Input: part model. Units: mm. Frame: model coordinates. A direction names the side the tool comes from. Round coordinates to 2 decimals unless told otherwise and drop trailing zeros. Write each loop counter-clockwise with the first axis right and the second up, starting at its lowest first coordinate (ties: lowest second). Pieces come first, ordered by that corner, then holes. Notation, with made-up numbers: (12.5, 46.5) -> (54.5, 46.5) arc R11 cw to (54.5, 55.5) -> close; hole circle Ø11 at (60, 10.25). An arc over 180 degrees is marked (long way). Write item = value, one per line. Start each with the question number.
```python
from build123d import *

# Parameters (mm, degrees)
SKETCH1_R           = 11.5
SKETCH1_R_2         = 1.5
SKETCH1_W           = 8.4
SKETCH1_H           = 8.4
BOSS_EXTRUDE1_DEPTH = 8.4


with BuildPart() as part:
    # Sketch1 → Boss-Extrude1 (new body)
    with BuildSketch(Plane(origin=(0, 0, 0), x_dir=(1, 0, 0), z_dir=(0, 1, 0))):
        with BuildLine():
            Line((-34.5, 26), (34.5, 26))
            ThreePointArc((34.5, 26), (36.621320344, 25.121320344), (37.5, 23))
            Line((37.5, 23), (37.5, -26))
            Line((37.5, -26), (23.5, -26))
            Line((23.5, -26), (23.5, -34))
            Line((23.5, -34), (15.5, -34))
            Line((15.5, -34), (15.5, -26))
            Line((15.5, -26), (2, -26))
            Line((2, -26), (2, -21.4))
            Line((2, -21.4), (3.5, -21.4))
            Line((3.5, -21.4), (3.5, -18.4))
            Line((3.5, -18.4), (2.260530911, -18.4))
            ThreePointArc((2.260530911, -18.4), (0, -11.1), (-2.260530911, -18.4))
            Line((-2.260530911, -18.4), (-3.5, -18.4))
            Line((-3.5, -18.4), (-3.5, -21.4))
            Line((-3.5, -21.4), (-2, -21.4))
            Line((-2, -21.4), (-2, -26))
            Line((-2, -26), (-15.5, -26))
            Line((-15.5, -26), (-15.5, -34))
            Line((-15.5, -34), (-23.5, -34))
            Line((-23.5, -34), (-23.5, -26))
            Line((-23.5, -26), (-37.5, -26))
            Line((-37.5, -26), (-37.5, 23))
            ThreePointArc((-37.5, 23), (-36.621320344, 25.121320344), (-34.5, 26))
        make_face()
        with Locations((0, 6)):
            Circle(SKETCH1_R, mode=Mode.SUBTRACT)
        with Locations((15.5, 21.5)):
            Circle(SKETCH1_R_2, mode=Mode.SUBTRACT)
        with Locations((-15.5, 21.5)):
            Circle(SKETCH1_R_2, mode=Mode.SUBTRACT)
        with Locations((15.5, -9.5)):
            Circle(SKETCH1_R_2, mode=Mode.SUBTRACT)
        with Locations((-15.5, -9.5)):
            Circle(SKETCH1_R_2, mode=Mode.SUBTRACT)
        with Locations((-30.1, 2)):
            Circle(SKETCH1_R_2, mode=Mode.SUBTRACT)
        with Locations((30.1, 2)):
            Circle(SKETCH1_R_2, mode=Mode.SUBTRACT)
        with Locations((-30.1, 14.2)):
            Rectangle(SKETCH1_W, SKETCH1_H, mode=Mode.SUBTRACT)
        with Locations((-30.1, -9.8)):
            Rectangle(SKETCH1_W, SKETCH1_H, mode=Mode.SUBTRACT)
        with Locations((30.1, -9.8)):
            Rectangle(SKETCH1_W, SKETCH1_H, mode=Mode.SUBTRACT)
        with Locations((30.1, 14.2)):
            Rectangle(SKETCH1_W, SKETCH1_H, mode=Mode.SUBTRACT)
    extrude(amount=BOSS_EXTRUDE1_DEPTH)


solid = part.part
```
1. Section D-D (z = -21.5). Output: boundary loops of the cut face in (x, y).
2. Section A-A (z = 27.5). Output: boundary loops of the cut face in (x, y), then the cut area to 3 significant figures.
3. Reachability of faces 1 (the flat face through (30, 4, 14)), 2 (the flat face through (23.5, 4, 30)), 3 (the flat face through (9, 4, 26)) from +Z, -Z, +X, -X, +Y, -Y: full face, straight path, thin tool, end or side. Return the list, or none.
4. Pin query (flat end, axial travel): P1, Ø1.4, axis at x = -3, y = 2, coming from the +Z side; P2, Ø2.5, axis at y = 2.5, z = 30.5, coming from the -X side. Return the tip coordinate at first contact, or that it passes through.
5. Mould query, pull axis X, two halves, no side actions, for faces 4 (the cylindrical face through (36.6, 4.14, -25.14)), 5 (the flat face through (34.3, 4, -14)), 6 (the flat face through (9, 8.4, 4)). Classes: pulls with the +X half, pulls with the -X half, needs draft (parallel to the pull), parting line crosses it, or undercut.
6. Line query: line 1 along Z through (x, y) = (-30.1, 3.75); line 2 along X through (y, z) = (6.5, 9.5); line 3 along Z through (x, y) = (-27, 1). Output: solid intervals per line, ascending.
7. Section C-C (x = 0). Output: boundary loops of the cut face in (y, z).
8. Section B-B (x = -30.1). Output: boundary loops of the cut face in (y, z), then the cut area to 3 significant figures.
Check sheet entries:
q1.outline = (-37.5, 0) -> (-17, 0) -> (-17, 8.4) -> (-37.5, 8.4) -> close; (-14, 0) -> (14, 0) -> (14, 8.4) -> (-14, 8.4) -> close; (17, 0) -> (37.5, 0) -> (37.5, 8.4) -> (17, 8.4) -> close
q2.outline = (-23.5, 0) -> (-15.5, 0) -> (-15.5, 8.4) -> (-23.5, 8.4) -> close; (15.5, 0) -> (23.5, 0) -> (23.5, 8.4) -> (15.5, 8.4) -> close
q2.area = 134 mm2
q3.face_1 = +Y, -Y
q3.face_2 = +Z, +X, +Y, -Y
q3.face_3 = +Z, +Y, -Y
q4.P1 = 26
q4.P2 = -23.5
q5.face_4 = pulls with the +X half
q5.face_5 = undercut
q5.face_6 = needs draft
q6.line_1 = -26 to -18.4, -10 to -3.5, -0.5 to 5.6, 14 to 26
q6.line_2 = -37.5 to -34.3, -25.9 to -17, -14 to 14, 17 to 25.9, 34.3 to 37.5
q6.line_3 = -26 to -18.4, -10 to 5.6, 14 to 26
q7.outline = (0, -26) -> (8.4, -26) -> (8.4, -17.5) -> (0, -17.5) -> close; (0, 5.5) -> (8.4, 5.5) -> (8.4, 11.1) -> (0, 11.1) -> close
q8.outline = (0, -26) -> (8.4, -26) -> (8.4, -18.4) -> (0, -18.4) -> close; (0, -10) -> (8.4, -10) -> (8.4, -3.5) -> (0, -3.5) -> close; (0, -0.5) -> (8.4, -0.5) -> (8.4, 5.6) -> (0, 5.6) -> close; (0, 14) -> (8.4, 14) -> (8.4, 26) -> (0, 26) -> close
q8.area = 270 mm2
